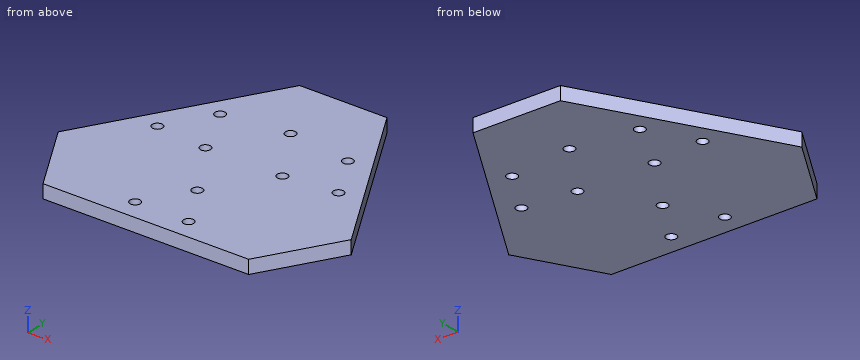
from build123d import *

# Parameters (mm, degrees)
BOSS_EXTRU_1_DEPTH      = 6.35
ENL_V_MAT_EXTRU_1_DEPTH = 136.945378124
D_GAGEMENT_M41_D        = 4.8
D_GAGEMENT_M43_D        = 4.8


with BuildPart() as part:
    # Esquisse1 → Boss.-Extru.1 (new body)
    with BuildSketch(Plane.XY):
        Polygon((-88.9, -51.326438931), (0, 102.652877862), (88.9, -51.326438931), align=None)
    extrude(amount=BOSS_EXTRU_1_DEPTH)

    # Esquisse2 → Enlèv. mat.-Extru.1 (cut, through all)
    with BuildSketch(Plane.XY.offset(6.35)):
        Polygon((-20.415865769, 67.291561069), (20.415865769, 67.291561069), (0, 102.652877862), align=None)
        Polygon((48.068268461, -51.326438931), (88.9, -51.326438931), (68.484134231, -15.965122138), align=None)
        Polygon((-68.484134231, -15.965122138), (-88.9, -51.326438931), (-48.068268461, -51.326438931), align=None)
    extrude(amount=-ENL_V_MAT_EXTRU_1_DEPTH, mode=Mode.SUBTRACT)

    # Dégagement M41 (through all)
    with Locations(Plane.XY.offset(6.35)):
        with Locations((12.5, -41.674438931), (-12.5, -41.674438931), (-42.341122803, 10.011901918), (-29.841122803, 31.662537013), (29.841122803, 31.662537013), (42.341122803, 10.011901918)):
            Hole(D_GAGEMENT_M41_D / 2)

    # Dégagement M43 (through all)
    with Locations(Plane.XY.offset(6.35)):
        with Locations((0, 35.6048), (0, -20.3952), (18, 7.6048), (-18, 7.6048)):
            Hole(D_GAGEMENT_M43_D / 2)


solid = part.part
Source: CAD feature listing. Evaluate the final solid. Frame: model axes, mm. Round coordinates to 2 decimals unless told otherwise and drop trailing zeros. Loops run counter-clockwise (first coordinate to the right, second up) from the corner with the lowest first, then second, coordinate; pieces in that order, holes last.
Q1. Section B-B, the plane z = 4.25. State how many separate pieces and enclosed holes the cut face has, plus the area to 3 significant figures.
Q2. Ray query, line 1 (Y direction, x = 0, z = 2.5); line 2 (X direction, y = 5.5, z = 3); line 3 (Y direction, x = -12.5, z = 2.75). Return the intervals inside material, ascending.
Q3. First-contact query: P1, Ø1.5, axis at y = 46.5, z = 2.5, coming from the -X side; P2, Ø3, axis at x = -43.5, z = 5.5, coming from the +Y side. Flat tips, straight axial feed; report the tip coordinate or a pass-through.
Q4. Section A-A, the plane x = -12.5. Return loops of the section in (y, z).
Q5. Section D-D, the plane x = -57. Return loops of the section in (y, z), plus the area to 3 significant figures.
Q6. Section C-C, the plane y = -7. Return loops of the section in (x, z), plus the area to 3 significant figures.
Solutions:
1. separate pieces: 1
1. enclosed holes: 10
1. area: 11,300 mm2
2. line 1: y = -51.33 to -22.8, -18 to 33.2, 38 to 67.29
2. line 2: x = -56.09 to -19.15, -16.85 to 16.85, 19.15 to 56.09
2. line 3: y = -51.33 to -44.07, -39.27 to 67.29
3. P1: stops at x = -32.85
3. P2: stops at y = 29.91
4. outline: (-51.33, 0) - (-44.07, 0) - (-44.07, 6.35) - (-51.33, 6.35) - close; (-39.27, 0) - (67.29, 0) - (67.29, 6.35) - (-39.27, 6.35) - close
5. outline: (-35.86, 0) - (3.93, 0) - (3.93, 6.35) - (-35.86, 6.35) - close
5. area: 253 mm2
6. outline: (-63.31, 0) - (63.31, 0) - (63.31, 6.35) - (-63.31, 6.35) - close
6. area: 804 mm2
